Geometry: final body of the model. Coordinates: model frame, mm. Give positions to 0.01 mm unless a question says otherwise; leave off trailing zeros. Write each loop counter-clockwise with the first axis right and the second up, starting at its lowest first coordinate (ties: lowest second). Pieces come first, ordered by that corner, then holes.
Q1. Pin query (flat end, axial travel): pin 1 Ø4 at (x, z) = (-9796.5, 202.5) entering from -Y; pin 2 Ø1.5 at (y, z) = (6730.5, 337) entering from +X; pin 3 Ø5 at (y, z) = (6706, 304) entering from +X. Return the tip coordinate at first contact, or that it passes through.
Q2. Section B-B (x = -9749). Return the cut outline in (y, z), plus the area to 3 significant figures.
Q3. Section C-C (y = 6918.5). Return the cut outline in (x, z), plus the area to 3 significant figures.
Q4. Section A-A (z = 68). Return the cut outline in (x, y), plus the area to 3 significant figures.
Q5. Line query: line 1 (Y direction, x = -9891, z = 62.5); line 2 (Y direction, x = -9858.5, z = 511.5); line 3 (X direction, y = 6825.5, z = 313.5). Output: solid intervals per line, ascending.
from build123d import *

# Parameters (mm, degrees)
EXTRUDE_1_DEPTH = 480
SCALE_1_SCALE   = 1.3


with BuildPart() as part:
    # 草图1 → 凸台-拉伸1 (new body)
    with BuildSketch(Plane.XY):
        with BuildLine():
            Line((-8158.198873592, 5112), (-7678.198873592, 5112))
            ThreePointArc((-7678.198873592, 5112), (-7531.058159836, 5261.115346452), (-7368.547684402, 5393.3126292))
            ThreePointArc((-7368.547684402, 5393.3126292), (-7256.775458313, 5468.670521429), (-7139.991111067, 5536))
            Line((-7139.991111067, 5536), (-7619.991111067, 5536))
            Line((-7619.991111067, 5536), (-8158.198873592, 5536))
            Line((-8158.198873592, 5536), (-8158.198873592, 5112))
        make_face()
    extrude(amount=EXTRUDE_1_DEPTH)


with BuildPart() as part_1:
    # 缩放比例1: scaled about (0, 0, 0)
    add(part.part.scale(SCALE_1_SCALE))


solid = part_1.part
Computed:
1. pin 1: stops at y = 6832.04
1. pin 2: stops at x = -9902.26
1. pin 3: stops at x = -9924.08
2. outline: (6876.21, 0) - (7196.8, 0) - (7196.8, 624) - (6876.21, 624) - close
2. area: 200,000 mm2
3. outline: (-10605.66, 0) - (-9699.01, 0) - (-9699.01, 624) - (-10605.66, 624) - close
3. area: 566,000 mm2
4. outline: (-10605.66, 6645.6) - (-9981.66, 6645.6) arc R2496 cw to (-9281.99, 7196.8) - (-10605.66, 7196.8) - close
4. area: 513,000 mm2
5. line 1: y = 6742.76 to 7196.8
5. line 2: y = 6775.19 to 7196.8
5. line 3: x = -10605.66 to -9805.6
